For this review, take the finished solid that the model builds, in its own axes (mm). A direction names the side the tool comes from. Coordinates: 2 decimals unless noted, no trailing zeros. Loops run counter-clockwise (first coordinate to the right, second up) from the corner with the lowest first, then second, coordinate; pieces in that order, holes last. Notation, with made-up numbers: M 1.25,71 L 54.25,71 A21 cw 54.25,105 Z; hole C -18.5,-7.5 d9. An arc over 180 degrees is marked long. Put each result on its own line as item: value.
```python
from build123d import *

# Parameters (mm, degrees)
SKETCH1_W                = 14
SKETCH1_H                = 28.85
SKETCH1_R                = 1.5
BOSS_EXTRUDE1_DEPTH      = 2.5
BOSS_EXTRUDE2_DEPTH      = 16.5
BOSS_EXTRUDE2_DEPTH_BACK = 5
SKETCH3_W                = 14
SKETCH3_H                = 2
SKETCH4_W                = 14
SKETCH4_H                = 2.5
BOSS_EXTRUDE3_DEPTH      = 15.6
SKETCH5_W                = 14
SKETCH5_H                = 2.5
BOSS_EXTRUDE4_DEPTH      = 21.5
SKETCH6_W                = 14
SKETCH6_H                = 6
BOSS_EXTRUDE5_DEPTH      = 16.5
BOSS_EXTRUDE6_DEPTH      = 14
FILLET2_R                = 5


with BuildPart() as part:
    # Sketch1 → Boss-Extrude1 (new body)
    with BuildSketch(Plane.XY):
        with Locations((7, 14.425)):
            Rectangle(SKETCH1_W, SKETCH1_H)
        with Locations((7, 26.35)):
            Circle(SKETCH1_R, mode=Mode.SUBTRACT)
        with Locations((7, 8.85)):
            Circle(SKETCH1_R, mode=Mode.SUBTRACT)
    extrude(amount=BOSS_EXTRUDE1_DEPTH)

    # Sketch3 → Boss-Extrude2 (add, two sides: drawn at the far end of the back side and taken through both)
    with BuildSketch(Plane.XY.offset(2.5).offset(-BOSS_EXTRUDE2_DEPTH_BACK)):
        with Locations((7, -1)):
            Rectangle(SKETCH3_W, SKETCH3_H)
    extrude(amount=BOSS_EXTRUDE2_DEPTH + BOSS_EXTRUDE2_DEPTH_BACK)

    # Sketch4 → Boss-Extrude3 (add)
    with BuildSketch(Plane(origin=(0, 28.85, 0), x_dir=(1, 0, 0), z_dir=(0, 1, 0))):
        with Locations((7, -1.25)):
            Rectangle(SKETCH4_W, SKETCH4_H)
    extrude(amount=BOSS_EXTRUDE3_DEPTH)

    # Sketch5 → Boss-Extrude4 (add)
    with BuildSketch(Plane.XY.offset(19)):
        with Locations((7, -1.25)):
            Rectangle(SKETCH5_W, SKETCH5_H)
    extrude(amount=-BOSS_EXTRUDE4_DEPTH)

    # Sketch6 → Boss-Extrude5 (add)
    with BuildSketch(Plane.XY.offset(2.5)):
        with Locations((7, 41.45)):
            Rectangle(SKETCH6_W, SKETCH6_H)
    extrude(amount=BOSS_EXTRUDE5_DEPTH)

    # Sketch7 → Boss-Extrude6 (add)
    with BuildSketch(Plane(origin=(14, 0, 0), x_dir=(0, 0, -1), z_dir=(1, 0, 0))):
        Polygon((-10.75, 38.45), (-2.5, 32.45), (-2.5, 38.45), align=None)
    extrude(amount=-BOSS_EXTRUDE6_DEPTH)

    # Fillet2
    fillet2_edges = [part.edges().sort_by_distance(p)[0] for p in [
        (7, 38.45, 10.75),
        (7, 32.45, 2.5),
    ]]
    fillet(fillet2_edges, radius=FILLET2_R)


solid = part.part
```
(1) For pin 1 (5 mm diameter, centred on x = 5.5, y = 21, fed in from -Z); pin 2 (4 mm diameter, centred on x = 7.5, y = 34.5, fed in from +Z); pin 3 (4 mm diameter, centred on x = 10, y = 13, fed in from +Z), all flat-tipped, find the tip position at first contact; note any pin that passes through.
Determined:
pin 1: stops at z = 0
pin 2: stops at z = 8.07
pin 3: stops at z = 2.5
(2) Wall thickness on line 1 along Y through (x, z) = (3.25, 17); line 2 along Z through (x, y) = (2, 8); line 3 along Y through (x, z) = (13, 5.25): over which ranges is each line inside the solid? List them lowest first. Write a range as [from, to].
Determined:
line 1: y = [-2.5, 0], [38.45, 44.45]
line 2: z = [0, 2.5]
line 3: y = [-2.5, 0], [34.45, 44.45]
(3) Add section C-C (z = 1.25). Write out the cut boundary in (x, y), plus the area to 3 significant figures.
Determined:
outline: M 0,-2.5 L 14,-2.5 L 14,44.45 L 0,44.45 Z; hole C 7,8.85 d3; hole C 7,26.35 d3
area: 643 mm^2
(4) Add section B-B (y = 26.35). Write out the cut boundary in (x, z), plus the area to 3 significant figures.
Determined:
outline: M 0,0 L 5.5,0 L 5.5,2.5 L 0,2.5 Z; M 8.5,0 L 14,0 L 14,2.5 L 8.5,2.5 Z
area: 27.5 mm^2
(5) Draft analysis for pull direction Y (two halves, no side actions). For faces 1 (the flat face through (7, -2.5, 8)), 2 (the flat face through (7, 41, 19)), 3 (the cylindrical face through (5.81, 25.44, 1.23)), state which applies: +Y half, -Y half, draft (parallel to the pull), parting line (faces both ways), or undercut.
Determined:
face 1: -Y half
face 2: draft
face 3: undercut
(6) Add section D-D (z = 17.25). Write out the cut boundary in (x, y), plus the area to 3 significant figures.
Determined:
outline: M 0,-2.5 L 14,-2.5 L 14,0 L 0,0 Z; M 0,38.45 L 14,38.45 L 14,44.45 L 0,44.45 Z
area: 119 mm^2
(7) Add section A-A (x = 7). Write out the cut boundary in (y, z).
Determined:
outline: M -2.5,-2.5 L 0,-2.5 L 0,0 L 7.35,0 L 7.35,2.5 L 0,2.5 L 0,19 L -2.5,19 Z; M 10.35,0 L 24.85,0 L 24.85,2.5 L 10.35,2.5 Z; M 27.85,0 L 44.45,0 L 44.45,19 L 38.45,19 L 38.45,12.38 A5 cw 37.49,9.44 L 33.95,4.56 A5 cw 29.9,2.5 L 27.85,2.5 Z
(8) Tool access review of faces 4 (the flat face through (7, -1, -2.5)), 5 (the flat face through (7, 0, -1)), 6 (the flat face through (7, 15, 2.5)): name each direction out of +Z, -Z, +X, -X, +Y, -Y from which nothing blocks a thin tool from reaching the whole face with its end or side.
Determined:
face 4: -Z, +X, -X, +Y, -Y
face 5: -Z, +X, -X, +Y
face 6: +Z, +X, -X
